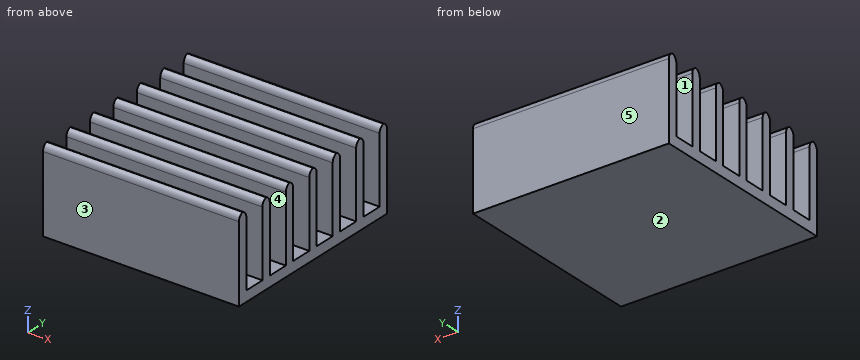
from build123d import *

# Parameters (mm, degrees)
BOSS_EXTRUDE1_DEPTH = 7
FILLET1_R           = 0.5


with BuildPart() as part:
    # Sketch1 → Boss-Extrude1 (new, symmetric)
    with BuildSketch(Plane(origin=(0, 0, 0), x_dir=(0, 0, -1), z_dir=(1, 0, 0))):
        Polygon((-6, 4.783333333), (-6, 4.083333333), (-0.75, 4.083333333), (-0.75, 2.566666667), (-6, 2.566666667), (-6, 1.866666667), (-0.75, 1.866666667), (-0.75, 0.35), (-6, 0.35), (-6, -0.35), (-0.75, -0.35), (-0.75, -1.866666667), (-6, -1.866666667), (-6, -2.566666667), (-0.75, -2.566666667), (-0.75, -4.083333333), (-6, -4.083333333), (-6, -4.783333333), (-0.75, -4.783333333), (-0.75, -6.3), (-6, -6.3), (-6, -7), (0, -7), (0, -6.3), (0, -4.783333333), (0, -4.083333333), (0, -2.566666667), (0, -1.866666667), (0, -0.35), (0, 0.35), (0, 1.866666667), (0, 2.566666667), (0, 4.083333333), (0, 4.783333333), (0, 6.3), (0, 7), (-6, 7), (-6, 6.3), (-0.75, 6.3), (-0.75, 4.783333333), align=None)
    extrude(amount=BOSS_EXTRUDE1_DEPTH, both=True)

    # Fillet1
    # the kernel refuses this fillet: 0.5 mm, written as the material it takes off along each edge
    with BuildSketch(Plane(origin=(-8.25, -7, 6), x_dir=(0, 0, -1), z_dir=(1, 0, 0)), Plane(origin=(-8.25, -6.3, 6), x_dir=(0, -1, 0), z_dir=(1, 0, 0)), Plane(origin=(-8.25, -4.783333333, 6), x_dir=(0, 0, -1), z_dir=(1, 0, 0)), Plane(origin=(-8.25, -4.083333333, 6), x_dir=(0, -1, 0), z_dir=(1, 0, 0)), Plane(origin=(-8.25, -2.566666667, 6), x_dir=(0, 0, -1), z_dir=(1, 0, 0)), Plane(origin=(-8.25, -1.866666667, 6), x_dir=(0, -1, 0), z_dir=(1, 0, 0)), Plane(origin=(-8.25, -0.35, 6), x_dir=(0, 0, -1), z_dir=(1, 0, 0)), Plane(origin=(-8.25, 0.35, 6), x_dir=(0, -1, 0), z_dir=(1, 0, 0)), Plane(origin=(-8.25, 1.866666667, 6), x_dir=(0, 0, -1), z_dir=(1, 0, 0)), Plane(origin=(-8.25, 2.566666667, 6), x_dir=(0, -1, 0), z_dir=(1, 0, 0)), Plane(origin=(-8.25, 6.3, 6), x_dir=(0, 0, -1), z_dir=(1, 0, 0)), Plane(origin=(-8.25, 7, 6), x_dir=(0, -1, 0), z_dir=(1, 0, 0))) as fillet1_piece_1:
        with BuildLine():
            CenterArc((FILLET1_R, FILLET1_R), FILLET1_R, 180, 90)
            Line((0, FILLET1_R), (0, 0))
            Line((0, 0), (FILLET1_R, 0))
        make_face()
    extrude(amount=16.5, mode=Mode.SUBTRACT)
    with BuildSketch(Plane(origin=(-8.25, 4.083333333, 6), x_dir=(0, 1, 0), z_dir=(1, 0, 0)), Plane(origin=(8.25, 4.783333333, 6), x_dir=(0, -1, 0), z_dir=(-1, 0, 0))) as fillet1_piece_2:
        with BuildLine():
            CenterArc((FILLET1_R, -FILLET1_R), FILLET1_R, 90, 90)
            Line((0, -FILLET1_R), (0, 0))
            Line((0, 0), (FILLET1_R, 0))
        make_face()
    extrude(amount=16.5, mode=Mode.SUBTRACT)


solid = part.part
Verification items for the finished model (mm, model axes). Face numbers are marked on the shaded views. A direction names the side the tool comes from. Round coordinates to 2 decimals unless told otherwise and drop trailing zeros. Order: outer loops, then holes, each group sorted by start corner. A loop starts at its lowest first (then second) coordinate and runs counter-clockwise, first axis right, second up.
1. Section check A-A on z = 2.25. Record the cut outline in (x, y).
Final values:
outline: (-7, -7) - (7, -7) - (7, -6.3) - (-7, -6.3) - close; (-7, -4.78) - (7, -4.78) - (7, -4.08) - (-7, -4.08) - close; (-7, -2.57) - (7, -2.57) - (7, -1.87) - (-7, -1.87) - close; (-7, -0.35) - (7, -0.35) - (7, 0.35) - (-7, 0.35) - close; (-7, 1.87) - (7, 1.87) - (7, 2.57) - (-7, 2.57) - close; (-7, 4.08) - (7, 4.08) - (7, 4.78) - (-7, 4.78) - close; (-7, 6.3) - (7, 6.3) - (7, 7) - (-7, 7) - close
2. Thickness scan on L1, parallel to Z at x = -4.75, y = -0.75; L2, parallel to Z at x = -2.25, y = -2. Record the ranges inside material, lowest first.
Final values:
L1: z = 0 to 0.75
L2: z = 0 to 5.84
3. Section check B-B on y = -3.25. Record the cut outline in (x, z).
Final values:
outline: (-7, 0) - (7, 0) - (7, 0.75) - (-7, 0.75) - close
4. Release check for a two-part mould opening along Y. For the marked faces 3, 4 and 5 record: +Y half, -Y half, draft (parallel to the pull), parting line (faces both ways), or undercut.
Final values:
face 3: -Y half
face 4: undercut
face 5: +Y half
5. Go/stop test with flat-tipped pins: P1, Ø0.5, axis at x = -1.5, y = -1, coming from the +Z side; P2, Ø2, axis at x = 3, y = 2, coming from the -Z side. Record where each tip stops, or that it passes through.
Final values:
P1: stops at z = 0.75
P2: stops at z = 0
6. Access from +Z, -Z, +X, -X, +Y, -Y to the whole of each face (thin tool, end or side, straight path). Record for the marked faces 1 and 2.
Final values:
face 1: +Z, +X, -X
face 2: -Z, +X, -X, +Y, -Y
